For this review, take the finished solid that the model builds, in its own axes (mm). A direction names the side the tool comes from. Round coordinates to 2 decimals unless told otherwise and drop trailing zeros. Order: outer loops, then holes, each group sorted by start corner. A loop starts at its lowest first (then second) coordinate and runs counter-clockwise, first axis right, second up. Notation, with made-up numbers: M 1.5,51 L 34.5,51 A10 ccw 34.5,58 Z; hole C 52.25,60 d1. An arc over 180 degrees is marked long. Answer in a Markdown table with one row per item. Add a question column.
```python
from build123d import *
from OCP.BRepFilletAPI import BRepFilletAPI_MakeChamfer

# Parameters (mm, degrees)
SKETCH1_W           = 80
SKETCH1_H           = 64
SKETCH1_W_2         = 40.7
SKETCH1_H_2         = 40
BOSS_EXTRUDE1_DEPTH = 15
SKETCH3_W           = 14
SKETCH3_H           = 11.1
SKETCH4_R           = 9.5
CUT_EXTRUDE2_DEPTH  = 88.458561616
SKETCH5_R           = 3
CUT_EXTRUDE3_DEPTH  = 77.948034413
SKETCH8_R           = 2.15
CUT_EXTRUDE6_DEPTH  = 54.37602458
FILLET1_R           = 20
CHAMFER1_SIZE       = 3
CHAMFER1_SIZE2      = 1.732050808
SKETCH9_W           = 12
SKETCH9_H           = 3
SKETCH10_W          = 24
SKETCH10_H          = 5.5
BOSS_EXTRUDE2_DEPTH = 8
BOSS_EXTRUDE3_START = 2
SKETCH12_W          = 24
SKETCH12_H          = 3.7
BOSS_EXTRUDE3_DEPTH = 6
BOSS_EXTRUDE4_DEPTH = 1.3
CHAMFER2_SIZE2      = 1.339745962
CHAMFER2_SIZE       = 5
CHAMFER3_SIZE       = 8
CHAMFER3_SIZE_2     = 4.618802154
CHAMFER4_SIZE       = 3
CHAMFER4_SIZE2      = 8.242432258


with BuildPart() as part:
    # Sketch1 → Boss-Extrude1 (new body)
    with BuildSketch(Plane(origin=(0, 0, 0), x_dir=(1, 0, 0), z_dir=(0, 1, 0))):
        Rectangle(SKETCH1_W, SKETCH1_H)
        Rectangle(SKETCH1_W_2, SKETCH1_H_2, mode=Mode.SUBTRACT)
    extrude(amount=BOSS_EXTRUDE1_DEPTH)

    # Sketch3 → Cut-Revolve1 (revolve, cut)
    with BuildSketch(Plane(origin=(0, 15, 0), x_dir=(1, 0, 0), z_dir=(0, 1, 0))):
        with Locations((27.35, -5.55)):
            Rectangle(SKETCH3_W, SKETCH3_H)
        with Locations((-27.35, -5.55)):
            Rectangle(SKETCH3_W, SKETCH3_H)
    revolve(axis=Axis((20.35, 15, 0), (1, 0, 0)), mode=Mode.SUBTRACT)

    # Sketch4 → Cut-Extrude2 (cut, through all)
    with BuildSketch(Plane(origin=(40, 0, 0), x_dir=(0, 0, -1), z_dir=(1, 0, 0))):
        with Locations((0, 15)):
            Circle(SKETCH4_R)
    extrude(amount=-CUT_EXTRUDE2_DEPTH, mode=Mode.SUBTRACT)

    # Sketch5 → Cut-Extrude3 (cut, through all)
    with BuildSketch(Plane.XY.offset(32)):
        with Locations((0, 15)):
            Circle(SKETCH5_R)
    extrude(amount=-CUT_EXTRUDE3_DEPTH, mode=Mode.SUBTRACT)

    # Sketch8 → Cut-Extrude6 (cut, through all)
    with BuildSketch(Plane(origin=(0, 15, 0), x_dir=(1, 0, 0), z_dir=(0, 1, 0))):
        with Locations(Location((24.5, 16.5, 0), (0, 0, 270))):
            Circle(SKETCH8_R)
        with Locations(Location((24.5, -16.5, 0), (0, 0, 270))):
            Circle(SKETCH8_R)
        with Locations(Location((-24.5, -16.5, 0), (0, 0, 270))):
            Circle(SKETCH8_R)
        with Locations(Location((-24.5, 16.5, 0), (0, 0, 270))):
            Circle(SKETCH8_R)
        with Locations(Location((9, -27, 0), (0, 0, 270))):
            Circle(SKETCH8_R)
        with Locations(Location((-9, -27, 0), (0, 0, 270))):
            Circle(SKETCH8_R)
        with Locations(Location((-9, 27, 0), (0, 0, 270))):
            Circle(SKETCH8_R)
        with Locations(Location((9, 27, 0), (0, 0, 270))):
            Circle(SKETCH8_R)
        with Locations(Location((-33, 16.5, 0), (0, 0, 270))):
            Circle(SKETCH8_R)
        with Locations(Location((-33, -16.5, 0), (0, 0, 270))):
            Circle(SKETCH8_R)
        with Locations(Location((33, -16.5, 0), (0, 0, 270))):
            Circle(SKETCH8_R)
        with Locations(Location((33, 16.5, 0), (0, 0, 270))):
            Circle(SKETCH8_R)
    extrude(amount=-CUT_EXTRUDE6_DEPTH, mode=Mode.SUBTRACT)

    # Fillet1
    fillet1_edges = [part.edges().sort_by_distance(p)[0] for p in [
        (-40, 7.5, -32),
        (40, 7.5, -32),
        (40, 7.5, 32),
        (-40, 7.5, 32),
    ]]
    fillet(fillet1_edges, radius=FILLET1_R)

    # Chamfer1: one chamfer whose edges measure the first distance from different faces: ONE call of the kernel's chamfer builder (chamfer() names one face for all edges)
    chamfer1_edges_1 = [part.edges().sort_by_distance(p)[0] for p in [
        (20.35, 3.9, 0),
    ]]
    chamfer1_side_1 = [part.faces().sort_by_distance(p)[0] for p in [
        (20.35, 0.427200187, 0),
    ]]
    chamfer1_edges_2 = [part.edges().sort_by_distance(p)[0] for p in [
        (-20.35, 3.9, 0),
    ]]
    chamfer1_side_2 = [part.faces().sort_by_distance(p)[0] for p in [
        (-20.35, 0.427200187, 0),
    ]]
    chamfer1 = BRepFilletAPI_MakeChamfer(part.part.solid().wrapped)
    for e in chamfer1_edges_1:
        chamfer1.Add(CHAMFER1_SIZE, CHAMFER1_SIZE2, e.wrapped, chamfer1_side_1[0].wrapped)  # the first distance lies on this face
    for e in chamfer1_edges_2:
        chamfer1.Add(CHAMFER1_SIZE, CHAMFER1_SIZE2, e.wrapped, chamfer1_side_2[0].wrapped)  # the first distance lies on this face
    add(Compound.cast(chamfer1.Shape()), mode=Mode.REPLACE)

    # Sketch9 → Cut-Revolve2 (revolve, cut)
    with BuildSketch(Plane(origin=(0, 15, 0), x_dir=(1, 0, 0), z_dir=(0, 1, 0))):
        with Locations((-6, -21.5)):
            Rectangle(SKETCH9_W, SKETCH9_H)
        with Locations((-6, 21.5)):
            Rectangle(SKETCH9_W, SKETCH9_H)
    revolve(axis=Axis((0, 15, -29.871415895), (0, 0, 1)), mode=Mode.SUBTRACT)

    # Sketch10 → Boss-Extrude2 (add)
    with BuildSketch(Plane.ZY.offset(40)):
        with Locations((0, 2.75)):
            Rectangle(SKETCH10_W, SKETCH10_H)
    extrude(amount=BOSS_EXTRUDE2_DEPTH)

    # Sketch12 → Boss-Extrude3 (add)
    with BuildSketch(Plane.ZY.offset(40).offset(BOSS_EXTRUDE3_START)):
        with Locations((0, 7.35)):
            Rectangle(SKETCH12_W, SKETCH12_H)
    extrude(amount=BOSS_EXTRUDE3_DEPTH)

    # Sketch13 → Boss-Extrude4 (add)
    with BuildSketch(Plane(origin=(0, 9.2, 0), x_dir=(1, 0, 0), z_dir=(0, 1, 0))):
        Polygon((-46.9, 2.2), (-46.9, 1.6), (-48, 1.6), (-48, 12), (-42, 12), (-42, -12), (-48, -12), (-48, -1.6), (-46.9, -1.6), (-46.9, -2.2), (-43.7, -2.2), (-43.7, 2.2), align=None)
    extrude(amount=BOSS_EXTRUDE4_DEPTH)

    # Chamfer2
    chamfer2_edges = [part.edges().sort_by_distance(p)[0] for p in [
        (-42, 10.5, 0),
    ]]
    chamfer2_side = [part.faces().sort_by_distance(p)[0] for p in [
        (-42, 10.473205081, 0),
    ]]
    chamfer(chamfer2_edges, length=CHAMFER2_SIZE - 0.0001, length2=CHAMFER2_SIZE2 - 0.0001, reference=chamfer2_side[0])  # a hair under: the kernel refuses the full size

    # Chamfer3
    chamfer3_edges_1 = [part.edges().sort_by_distance(p)[0] for p in [
        (-48, 5.25, 12),
    ]]
    chamfer3_side_1 = [part.faces().sort_by_distance(p)[0] for p in [
        (-47.907623957, 5.25, 12),
    ]]
    chamfer3_edges_2 = [part.edges().sort_by_distance(p)[0] for p in [
        (-48, 5.25, -12),
    ]]
    chamfer3_side_2 = [part.faces().sort_by_distance(p)[0] for p in [
        (-47.907623957, 5.25, -12),
    ]]
    chamfer3 = BRepFilletAPI_MakeChamfer(part.part.solid().wrapped)
    for e in chamfer3_edges_1:
        chamfer3.Add(CHAMFER3_SIZE - 0.0001, CHAMFER3_SIZE_2 - 0.0001, e.wrapped, chamfer3_side_1[0].wrapped)
    for e in chamfer3_edges_2:
        chamfer3.Add(CHAMFER3_SIZE - 0.0001, CHAMFER3_SIZE_2 - 0.0001, e.wrapped, chamfer3_side_2[0].wrapped)
    add(Compound.cast(chamfer3.Shape()), mode=Mode.REPLACE)  # a hair under: the kernel refuses the full size

    # Chamfer4
    chamfer4_edges = [part.edges().sort_by_distance(p)[0] for p in [
        (-48, 0, 0),
    ]]
    chamfer4_side = [part.faces().sort_by_distance(p)[0] for p in [
        (-40.00005, 0, 10.911882359),
    ]]
    chamfer(chamfer4_edges, length=CHAMFER4_SIZE, length2=CHAMFER4_SIZE2, reference=chamfer4_side[0])


solid = part.part
```
1. Consider section A-A on z = -27. Write out the cut boundary in (x, y), plus the area to 3 significant figures.
2. Consider section B-B on x = 9. Write out the cut boundary in (y, z).
3. To check wall thickness, follow probe 1 along Z at (x, y) = (14.5, 11); probe 2 along Z at (x, y) = (30, 8); probe 3 along Z at (x, y) = (25.5, 8.75). State the ranges of each line that lie inside material, in increasing order. Write a range as [from, to].
4. For faces 5 (the flat face through (20.35, 0.7, 0.3)), 6 (the cylindrical face through (37.215, 5.502, 0.209)), 7 (the flat face through (0, 9, -23)), list the 3-axis set-ups (+Z, -Z, +X, -X, +Y, -Y) from which the entire face can be reached by the end or side of a thin tool; tool diameter is ignored.
5. Clearance check with flat-ended pins moving along their axes: pin 1 Ø2 at (y, z) = (11, -21.5) entering from +X; pin 2 Ø1 at (y, z) = (11.5, -23) entering from +X; pin 3 Ø0.6 at (x, y) = (-47.5, 10) entering from -Z. State where each tip first meets the part, or that it passes through.
6. The part is to be moulded in two halves that separate along Z. For faces 1 (the flat face through (-44.056, 5.323, -9.658)), 2 (the flat face through (-45.6, 10.5, -2.4)), 3 (the conical face through (22, 3.76, 0.25)), 4 (the cylindrical face through (-26.6, 7.6, 16.03)), say which applies: pulls with the +Z half, pulls with the -Z half, needs draft (parallel to the pull), parting line crosses it, or undercut.
7. Consider section C-C on z = -16.5. Write out the cut boundary in (x, y).
8. Consider section D-D on x = -24.5. Write out the cut boundary in (y, z), plus the area to 3 significant figures.
Solved:
| question | item | result |
|---|---|---|
| 1 | outline | M -33.23,0 L -11.15,0 L -11.15,15 L -33.23,15 Z; M -6.85,0 L 6.85,0 L 6.85,15 L 3,15 A3 cw -3,15 L -6.85,15 Z; M 11.15,0 L 33.23,0 L 33.23,15 L 11.15,15 Z |
| 1 | area | 854 mm^2 |
| 2 | outline | M 0,-32 L 15,-32 L 15,-29.15 L 0,-29.15 Z; M 0,-24.85 L 15,-24.85 L 15,-23 L 7.06,-23 L 7.06,-20 L 0,-20 Z; M 0,20 L 7.06,20 L 7.06,23 L 15,23 L 15,24.85 L 0,24.85 Z; M 0,29.15 L 15,29.15 L 15,32 L 0,32 Z |
| 3 | probe 1 | z = [-32, -20], [20, 32] |
| 3 | probe 2 | z = [-29.32, -8.61], [8.61, 29.32] |
| 3 | probe 3 | z = [-31.23, -18.4], [-14.6, -9.17], [9.17, 14.6], [18.4, 31.23] |
| 4 | face 5 | +Y, -Y |
| 4 | face 6 | +X, +Y |
| 4 | face 7 | +Y |
| 5 | pin 1 | stops at x = 38.1 |
| 5 | pin 2 | stops at x = 37.02 |
| 5 | pin 3 | stops at z = -7.84 |
| 6 | face 1 | pulls with the -Z half |
| 6 | face 2 | needs draft |
| 6 | face 3 | undercut |
| 6 | face 4 | undercut |
| 7 | outline | M -39.49,0 L -35.15,0 L -35.15,15 L -39.49,15 Z; M -30.85,0 L -26.65,0 L -26.65,15 L -30.85,15 Z; M -22.35,0 L -20.35,0 L -20.35,15 L -22.35,15 Z; M 20.35,0 L 22.35,0 L 22.35,15 L 20.35,15 Z; M 26.65,0 L 30.85,0 L 30.85,15 L 26.65,15 Z; M 35.15,0 L 39.49,0 L 39.49,15 L 35.15,15 Z |
| 8 | outline | M 0,-31.49 L 15,-31.49 L 15,-18.65 L 0,-18.65 Z; M 0,-14.35 L 15,-14.35 L 15,-11.1 A11.1 cw 15,11.1 L 15,14.35 L 0,14.35 Z; M 0,18.65 L 15,18.65 L 15,31.49 L 0,31.49 Z |
| 8 | area | 622 mm^2 |
